Autodesk Inventor part; units mm, degrees
ref_plane "YZ Plane" through (0, 0, 0) normal (1, 0, 0) x (0, 1, 0)
ref_plane "XZ Plane" through (0, 0, 0) normal (0, 1, 0) x (-1, 0, 0)
ref_plane "XY Plane" through (0, 0, 0) normal (0, 0, 1) x (1, 0, 0)
sketch "Эскиз1" plane through (0, 0, 0) normal (0, 1, 0) x (-1, 0, 0)
  circle A0 centre (0, 0) radius 6
  dimension "d0" = 12
extrude "Выдавливание1" add sketch "Эскиз1" along normal blind 60
thread "Резьба1"
sketch "Эскиз2" plane through (0, 0, 0) normal (0, -1, 0) x (1, 0, 0)
  line L0 (9.5, 5.4848) -> (9.5, -5.4848)
  line L1 (9.5, -5.4848) -> (0, -10.9697)
  line L2 (0, -10.9697) -> (-9.5, -5.4848)
  line L3 (-9.5, -5.4848) -> (-9.5, 5.4848)
  line L4 (-9.5, 5.4848) -> (0, 10.9697)
  line L5 (0, 10.9697) -> (9.5, 5.4848)
  line L6 (0, -15.3575) -> (0, 15.3575) construction
  point P0 (0, 0)
  point P1 (0, 0)
  dimension "d5" = 19
extrude "Выдавливание2" add sketch "Эскиз2" along normal blind 7.5
sketch "Эскиз3" plane through (0, -7.5, 0) normal (0, -1, 0) x (1, 0, 0)
  circle A0 centre (0, 0) radius 3
  dimension "d8" = 6
extrude "Выдавливание3" cut sketch "Эскиз3" against normal blind 20
sketch "Эскиз4" plane through (9.5, 0, 5.4848) normal (1, 0, 0) x (0, 0, -1)
  circle A0 centre (5.4848, -3.75) radius 2
  line L0 (10.9697, -7.5) -> (0, -7.5)
  point P0 (5.4848, 0)
  dimension "d11" = 4
  dimension "d12" = 3.75
extrude "Выдавливание4" cut sketch "Эскиз4" against normal blind 8.5
thread "Резьба2"
chamfer "Фаска1" distance 1 angle 45 1 edges at (6, 60, 0)
properties part number "KB33-046-002-002 - Втулка"
Check sheet for the modelled part. Datum: model origin and axes. Units: mm. A direction names the side the tool comes from. Give positions to 0.01 mm unless a question says otherwise; leave off trailing zeros. Loops run counter-clockwise (first coordinate to the right, second up) from the corner with the lowest first, then second, coordinate; pieces in that order, holes last. Notation, with made-up numbers: M 76,13.5 L 91,13.5 A32 cw 91,50.5 Z; hole C -0.75,-0.75 d8. An arc over 180 degrees is marked long. Answer as a JSON object with one key per item and string values. Group by question number.
Q1. Material ranges on line 1 along X through (y, z) = (9, 0.25); line 2 along Y through (x, z) = (8.25, 0); line 3 along Y through (x, z) = (1, -1.5), recorded low to high. Write a range as [from, to].
Q2. Cross-section at C-C on z = -9. Record the cut outline in (x, y).
Q3. Access from +Z, -Z, +X, -X, +Y, -Y to the whole of each face (thin tool, end or side, straight path). Record for faces 1 (the cylindrical face through (-3, 2, 0)), 2 (the flat face through (0, 60, 0)), 3 (the flat face through (-4, 0, -5)).
Q4. Cross-section at D-D on x = -8.5. Record the cut outline in (y, z), then the cut area to 3 significant figures.
Q5. Release check for a two-part mould opening along Z. For faces 4 (the flat face through (0, 12.5, 0)), 5 (the cylindrical face through (6, 29, 0)), 6 (the cylindrical face through (5.9, -3.7, 2)), 7 (the flat face through (4.8, -3.7, -8.2)) record: released by +Z, released by -Z, zero draft, split by the parting line, or undercut.
Q6. Cross-section at B-B on y = -3.75. Record the cut outline in (x, z).
Q7. Go/stop test with flat-tipped pins: P1, Ø1.8, axis at x = 0.5, z = 0, coming from the -Y side; P2, Ø3, axis at x = 5, y = 51, coming from the +Z side; P3, Ø5, axis at y = 22.5, z = -5, coming from the -X side. Record where each tip stops, or that it passes through.
Q8. Cross-section at A-A on z = 0. Record the cut outline in (x, y), then the cut area to 4 significant figures.
Evaluation:
{
 "1": {"line 1": "x = [-5.99, -2.99], [2.99, 5.99]", "line 2": "y = [-7.5, -5.75], [-1.75, 0]", "line 3": "y = [12.5, 60]"},
 "2": {"outline": "M -3.41,-7.5 L 3.41,-7.5 L 3.41,0 L -3.41,0 Z"},
 "3": {"face 1": "-Y", "face 2": "+Z, -Z, +X, -X, +Y", "face 3": "+Y"},
 "4": {"outline": "M -7.5,-6.06 L 0,-6.06 L 0,6.06 L -7.5,6.06 Z", "area": "90.9 mm2"},
 "5": {"face 4": "undercut", "face 5": "split by the parting line", "face 6": "undercut", "face 7": "released by -Z"},
 "6": {"outline": "M -9.5,-5.48 L 0,-10.97 L 9.5,-5.48 L 9.5,-2 L 2.24,-2 A3 cw long 2.24,2 L 9.5,2 L 9.5,5.48 L 0,10.97 L -9.5,5.48 Z"},
 "7": {"P1": "stops at y = 12.5", "P2": "stops at z = 4.87", "P3": "stops at x = -5.45"},
 "8": {"outline": "M -9.5,-7.5 L -3,-7.5 L -3,12.5 L 3,12.5 L 3,-1.75 L 9.5,-1.75 L 9.5,0 L 6,0 L 6,59 L 5,60 L -5,60 L -6,59 L -6,0 L -9.5,0 Z; M 3,-7.5 L 9.5,-7.5 L 9.5,-5.75 L 3,-5.75 Z", "area": "715.5 mm2"}
}
